from build123d import *

# Parameters (mm, degrees)
CROQUIS1_W              = 80
CROQUIS1_H              = 74
SALIENTE_EXTRUIR1_DEPTH = 20
CROQUIS3_R              = 4
CORTAR_EXTRUIR2_DEPTH   = 25
CROQUIS4_R              = 4
CORTAR_EXTRUIR3_DEPTH   = 30


with BuildPart() as part:
    # Croquis1 → Saliente-Extruir1 (new body)
    with BuildSketch(Plane(origin=(0, 0, 0), x_dir=(0, 0, -1), z_dir=(1, 0, 0))):
        Rectangle(CROQUIS1_W, CROQUIS1_H)
    extrude(amount=-SALIENTE_EXTRUIR1_DEPTH)

    # Croquis3 → Cortar-Extruir2 (cut)
    with BuildSketch(Plane(origin=(0, 37, 0), x_dir=(1, 0, 0), z_dir=(0, 1, 0))):
        with Locations(Location((-10, -18, 0), (0, 0, 270))):
            Circle(CROQUIS3_R)
        with Locations(Location((-10, 18, 0), (0, 0, 270))):
            Circle(CROQUIS3_R)
    extrude(amount=-CORTAR_EXTRUIR2_DEPTH, mode=Mode.SUBTRACT)

    # Croquis4 → Cortar-Extruir3 (cut)
    with BuildSketch(Plane.XZ.offset(37)):
        with Locations(Location((-10, 30, 0), (0, 0, 270))):
            Circle(CROQUIS4_R)
        with Locations(Location((-10, -30, 0), (0, 0, 270))):
            Circle(CROQUIS4_R)
    extrude(amount=-CORTAR_EXTRUIR3_DEPTH, mode=Mode.SUBTRACT)


solid = part.part
The model under review builds one solid part; all positions refer to its coordinate system, in mm. A direction names the side the tool comes from. Give positions to 0.01 mm unless a question says otherwise; leave off trailing zeros. Loops run counter-clockwise (first coordinate to the right, second up) from the corner with the lowest first, then second, coordinate; pieces in that order, holes last. Notation, with made-up numbers: (75, -10) -> (120, -10) arc R28 ccw to (120, 18) -> close; hole circle Ø9 at (51, 70.25). An arc over 180 degrees is marked (long way). Answer as a JSON object with one key per item and string values. Group by question number.
Q1. Wall thickness on line 1 along X through (y, z) = (-20.75, -30); line 2 along X through (y, z) = (-16, 31.5); line 3 along Y through (x, z) = (-7.25, -28): over which ranges is each line inside the solid? List them lowest first.
Q2. Tool access review of faces 1 (the flat face through (-10, -7, 30)), 2 (the cylindrical face through (-12.4, 24.7, 14.8)), 3 (the flat face through (-10, -37, 1)): name each direction out of +Z, -Z, +X, -X, +Y, -Y from which nothing blocks a thin tool from reaching the whole face with its end or side.
Q3. Insertion check: pin 1 (6.5 mm diameter, centred on x = -10, z = 18, fed in from +Y); pin 2 (5 mm diameter, centred on x = -10, z = 30, fed in from -Y). Each pin has a flat end and moves straight along its axis. Give the tip position at first contact, or say it passes through.
Q4. Take a section at B-B (y = -23). Write out the cut boundary in (x, z), plus the area to 3 significant figures.
Q5. Take a section at C-C (x = -10). Write out the cut boundary in (y, z), plus the area to 3 significant figures.
Q6. Draft analysis for pull direction X (two halves, no side actions). For faces 4 (the cylindrical face through (-12.4, -22.2, -26.8)), 5 (the cylindrical face through (-12.4, -22.2, 33.2)), 6 (the flat face through (0, 1, 1)), 7 (the flat face through (-10, 37, 1)), state which applies: pulls with the +X half, pulls with the -X half, needs draft (parallel to the pull), parting line crosses it, or undercut.
Q7. Take a section at D-D (z = 18). Write out the cut boundary in (x, y), plus the area to 3 significant figures.
Q8. Take a section at A-A (z = 30). Write out the cut boundary in (x, y), plus the area to 3 significant figures.
Answer below:
{
 "1": {"line 1": "x = -20 to -14, -6 to 0", "line 2": "x = -20 to -13.71, -6.29 to 0", "line 3": "y = -7 to 37"},
 "2": {"face 1": "-Y", "face 2": "+Y", "face 3": "+Z, -Z, +X, -X, -Y"},
 "3": {"pin 1": "stops at y = 12", "pin 2": "stops at y = -7"},
 "4": {"outline": "(-20, -40) -> (0, -40) -> (0, 40) -> (-20, 40) -> close; hole circle Ø8 at (-10, -30); hole circle Ø8 at (-10, 30)", "area": "1,500 mm2"},
 "5": {"outline": "(-37, -40) -> (37, -40) -> (37, -22) -> (12, -22) -> (12, -14) -> (37, -14) -> (37, 14) -> (12, 14) -> (12, 22) -> (37, 22) -> (37, 40) -> (-37, 40) -> (-37, 34) -> (-7, 34) -> (-7, 26) -> (-37, 26) -> (-37, -26) -> (-7, -26) -> (-7, -34) -> (-37, -34) -> close", "area": "5,040 mm2"},
 "6": {"face 4": "undercut", "face 5": "undercut", "face 6": "pulls with the +X half", "face 7": "needs draft"},
 "7": {"outline": "(-20, -37) -> (0, -37) -> (0, 37) -> (-6, 37) -> (-6, 12) -> (-14, 12) -> (-14, 37) -> (-20, 37) -> close", "area": "1,280 mm2"},
 "8": {"outline": "(-20, -37) -> (-14, -37) -> (-14, -7) -> (-6, -7) -> (-6, -37) -> (0, -37) -> (0, 37) -> (-20, 37) -> close", "area": "1,240 mm2"}
}
